Design review of the part built by this model. Coordinates are the model's own, in mm. A direction names the side the tool comes from. Round coordinates to 2 decimals unless told otherwise and drop trailing zeros. Order: outer loops, then holes, each group sorted by start corner. A loop starts at its lowest first (then second) coordinate and runs counter-clockwise, first axis right, second up.
from build123d import *

# Parameters (mm, degrees)
BOSS_EXTRUDE1_DEPTH       = 15.875
BOSS_EXTRUDE1_START       = -16.6878
BOSS_EXTRUDE1_2_OUTLINE_W = 13.242442679
BOSS_EXTRUDE1_2_OUTLINE_H = 1.4224
BOSS_EXTRUDE1_2_DEPTH     = 16.6878
BOSS_EXTRUDE2_START       = 15.875
BOSS_EXTRUDE2_DEPTH       = 15.875
SKETCH3_W                 = 13.242442679
SKETCH3_H                 = 1.4224
BOSS_EXTRUDE3_DEPTH       = 7.5311
SKETCH4_W                 = 13.242442679
SKETCH4_H                 = 1.4224
BOSS_EXTRUDE4_DEPTH       = 7.5311
CUT_EXTRUDE1_DEPTH        = 38.226845626
CUT_EXTRUDE2_DEPTH        = 38.226845626
CUT_EXTRUDE3_DEPTH        = 38.226845626
CUT_EXTRUDE4_DEPTH        = 38.226845626
SKETCH9_W                 = 4.6228
SKETCH9_H                 = 4.6228
CUT_EXTRUDE5_DEPTH        = 38.429132244
SKETCH10_W                = 4.6228
SKETCH10_H                = 4.6228
CUT_EXTRUDE6_DEPTH        = 38.429132244
SKETCH11_W                = 4.6228
SKETCH11_H                = 4.6228
CUT_EXTRUDE7_DEPTH        = 38.429132244
SKETCH12_W                = 4.6228
SKETCH12_H                = 4.6228
CUT_EXTRUDE8_DEPTH        = 38.429132244
SKETCH13_W                = 4.6228
SKETCH13_H                = 4.6228
CUT_EXTRUDE9_DEPTH        = 38.226845626
DRAFT1_ANGLE              = 45
DRAFT2_ANGLE              = 45
CHAMFER1_SIZE             = 2.24506403
SKETCH14_R                = 2.413
CUT_EXTRUDE10_DEPTH       = 2.54
LPATTERN1_COUNT           = 5
LPATTERN1_PITCH           = 12.7


with BuildPart() as part:
    # Boss-Extrude1: read off the stored shape, not the designer's step
    # Boss-Extrude1 outline → Boss-Extrude1 (new body)
    with BuildSketch(Plane(origin=(0, 0, -8.3439), x_dir=(-1, 0, 0), z_dir=(0, 0, -1))):
        with BuildLine():
            ThreePointArc((15.875, 0), (17.379950004, 5.616549878), (13.26835013, 1.504950004))
            Line((13.26835013, 1.504950004), (14.500184664, 2.216150004))
            ThreePointArc((14.500184664, 2.216150004), (16.668750004, 4.384715344), (15.875, 1.4224))
            Line((15.875, 1.4224), (-3.175, 1.4224))
            Line((-3.175, 1.4224), (-3.175, 0))
            Line((-3.175, 0), (15.875, 0))
        make_face()
    extrude(amount=BOSS_EXTRUDE1_DEPTH)

    # Boss-Extrude1 2 outline → Boss-Extrude1 2 (add)
    with BuildSketch(Plane(origin=(0, 0, -8.3439), x_dir=(-1, 0, 0), z_dir=(0, 0, -1)).offset(BOSS_EXTRUDE1_START)):
        with Locations((3.44622134, 0.7112)):
            Rectangle(BOSS_EXTRUDE1_2_OUTLINE_W, BOSS_EXTRUDE1_2_OUTLINE_H)
    extrude(amount=BOSS_EXTRUDE1_2_DEPTH)

    # Sketch2 → Boss-Extrude2 (add)
    with BuildSketch(Plane.XY.offset(8.3439).offset(BOSS_EXTRUDE2_START)):
        with BuildLine():
            Line((3.175, -6e-09), (-15.875, -6e-09))
            ThreePointArc((-15.875, -6e-09), (-17.379950004, 5.616549873), (-13.26835013, 1.504949999))
            Line((-13.26835013, 1.504949999), (-14.500184664, 2.216149999))
            ThreePointArc((-14.500184664, 2.216149999), (-16.668750004, 4.384715339), (-15.875, 1.422399994))
            Line((-15.875, 1.422399994), (3.175, 1.422399994))
            Line((3.175, 1.422399994), (3.175, -6e-09))
        make_face()
    extrude(amount=-BOSS_EXTRUDE2_DEPTH)

    # Sketch3 → Boss-Extrude3 (add)
    with BuildSketch(Plane(origin=(0, 0, -24.2189), x_dir=(-1, 0, 0), z_dir=(0, 0, -1))):
        with Locations((3.44622134, 0.7112)):
            Rectangle(SKETCH3_W, SKETCH3_H)
    extrude(amount=BOSS_EXTRUDE3_DEPTH)

    # Sketch4 → Boss-Extrude4 (add)
    with BuildSketch(Plane.XY.offset(24.2189)):
        with Locations((-3.44622134, 0.7112)):
            Rectangle(SKETCH4_W, SKETCH4_H)
    extrude(amount=BOSS_EXTRUDE4_DEPTH)

    # Sketch5 → Cut-Extrude1 (cut, through all)
    with BuildSketch(Plane(origin=(0, 1.4224, 0), x_dir=(-1, 0, 0), z_dir=(0, 1, 0))):
        Polygon((-3.175, -16.80493597), (-3.175, -21.29506403), (1.315128061, -16.80493597), align=None)
    extrude(amount=-CUT_EXTRUDE1_DEPTH, mode=Mode.SUBTRACT)

    # Sketch6 → Cut-Extrude2 (cut, through all)
    with BuildSketch(Plane(origin=(0, 1.4224, 0), x_dir=(-1, 0, 0), z_dir=(0, 1, 0))):
        Polygon((-3.175, -4.10493597), (-3.175, -8.59506403), (1.315128061, -8.59506403), align=None)
    extrude(amount=-CUT_EXTRUDE2_DEPTH, mode=Mode.SUBTRACT)

    # Sketch7 → Cut-Extrude3 (cut, through all)
    with BuildSketch(Plane(origin=(0, 1.4224, 0), x_dir=(-1, 0, 0), z_dir=(0, 1, 0))):
        Polygon((-3.175, 8.59506403), (-3.175, 4.10493597), (1.315128061, 8.59506403), align=None)
    extrude(amount=-CUT_EXTRUDE3_DEPTH, mode=Mode.SUBTRACT)

    # Sketch8 → Cut-Extrude4 (cut, through all)
    with BuildSketch(Plane(origin=(0, 1.4224, 0), x_dir=(-1, 0, 0), z_dir=(0, 1, 0))):
        Polygon((-3.175, 21.29506403), (-3.175, 16.80493597), (1.315128061, 16.80493597), align=None)
    extrude(amount=-CUT_EXTRUDE4_DEPTH, mode=Mode.SUBTRACT)

    # Sketch9 → Cut-Extrude5 (cut, through all)
    with BuildSketch(Plane.XZ):
        with Locations((-3.175, 25.4)):
            Rectangle(SKETCH9_W, SKETCH9_H)
    extrude(amount=-CUT_EXTRUDE5_DEPTH, mode=Mode.SUBTRACT)

    # Sketch10 → Cut-Extrude6 (cut, through all)
    with BuildSketch(Plane.XZ):
        with Locations((-3.175, 12.7)):
            Rectangle(SKETCH10_W, SKETCH10_H)
    extrude(amount=-CUT_EXTRUDE6_DEPTH, mode=Mode.SUBTRACT)

    # Sketch11 → Cut-Extrude7 (cut, through all)
    with BuildSketch(Plane.XZ):
        with Locations((-3.175, 0)):
            Rectangle(SKETCH11_W, SKETCH11_H)
    extrude(amount=-CUT_EXTRUDE7_DEPTH, mode=Mode.SUBTRACT)

    # Sketch12 → Cut-Extrude8 (cut, through all)
    with BuildSketch(Plane.XZ):
        with Locations((-3.175, -12.7)):
            Rectangle(SKETCH12_W, SKETCH12_H)
    extrude(amount=-CUT_EXTRUDE8_DEPTH, mode=Mode.SUBTRACT)

    # Sketch13 → Cut-Extrude9 (cut, through all)
    with BuildSketch(Plane(origin=(0, 1.4224, 0), x_dir=(-1, 0, 0), z_dir=(0, 1, 0))):
        with Locations((3.175, -25.4)):
            Rectangle(SKETCH13_W, SKETCH13_H)
    extrude(amount=-CUT_EXTRUDE9_DEPTH, mode=Mode.SUBTRACT)

    # Draft1
    draft1_faces = [part.faces().sort_by_distance(p)[0] for p in [
        (0.92993597, 0.7112, -8.59506403),
        (0.92993597, 0.711199999, -16.80493597),
    ]]
    draft(draft1_faces, Plane(origin=(3.175, 0, 31.75), x_dir=(0, 0, 1), z_dir=(1, 0, 0)), DRAFT1_ANGLE)

    # Draft2
    draft2_faces = [part.faces().sort_by_distance(p)[0] for p in [
        (0.92993597, 0.7112, 16.80493597),
        (0.92993597, 0.711199997, 8.59506403),
    ]]
    draft(draft2_faces, Plane(origin=(3.175, 0, 31.75), x_dir=(0, 0, 1), z_dir=(1, 0, 0)), DRAFT2_ANGLE)

    # Chamfer1
    chamfer1_edges = [part.edges().sort_by_distance(p)[0] for p in [
        (3.175, 0.7112, 31.75),
        (-10.067442679, 0.7112, 31.75),
        (3.175, 0.7112, -31.75),
        (-10.067442679, 0.7112, -31.75),
    ]]
    chamfer(chamfer1_edges, length=CHAMFER1_SIZE)

    # Sketch14 → Cut-Extrude10 (cut)
    with BuildSketch(Plane(origin=(0, 1.4224, 0), x_dir=(1, 0, 0), z_dir=(0, 1, 0))):
        with Locations((-3.175, -25.4)):
            Circle(SKETCH14_R)
    cut_extrude10 = extrude(amount=-CUT_EXTRUDE10_DEPTH, mode=Mode.SUBTRACT)

    # LPattern1: Cut-Extrude10 ×5
    with Locations(*[(0, 0, -i * LPATTERN1_PITCH) for i in range(1, LPATTERN1_COUNT)]):
        add(cut_extrude10, mode=Mode.SUBTRACT)


solid = part.part
1) To check wall thickness, follow line 1 along Z through (x, y) = (-2, 0.5); line 2 along Z through (x, y) = (-17.75, 2.5); line 3 along Y through (x, z) = (-1.5, 18.5). State the ranges of each line that lie inside material, in increasing order.
Results:
line 1: z = -31.75 to -27.71, -23.09 to -15.01, -10.39 to -2.31, 2.31 to 10.39, 15.01 to 23.09, 27.71 to 31.75
line 2: z = -24.22 to -8.34, 8.34 to 24.22
line 3: y = 0 to 1.42
2) Clearance check with flat-ended pins moving along their axes: P1, Ø3, axis at y = 1, z = -2, coming from the -X side; P2, Ø1.1, axis at y = 0.5, z = 14, coming from the -X side; P3, Ø3, axis at x = -12, z = 2, coming from the +Y side; P4, Ø1.6, axis at y = 0.5, z = 11.5, coming from the -X side. State where each tip first meets the part, or that it passes through.
Results:
P1: stops at x = -10.07
P2: stops at x = -18.16
P3: passes through
P4: stops at x = -18.35
3) For faces 1 (the face through (3.175, 1, -25)), 2 (the face through (2.04, 0.72, 7.46)), 3 (the face through (-13.88, 1.86, -16.17)), 4 (the face through (-0.864, 1, 1)), list the 3-axis set-ups (+Z, -Z, +X, -X, +Y, -Y) from which the entire face can be reached by the end or side of a thin tool; tool diameter is ignored.
Results:
face 1: +Z, -Z, +X, +Y, -Y
face 2: +X, +Y, -Y
face 3: +Z, -Z
face 4: +Y, -Y
4) Take a section at C-C on y = 4. Give the boundary of the cut face in (x, z), plus the area to 3 significant figures.
Results:
outline: (-18.72, -24.22) - (-17.12, -24.22) - (-17.12, -8.34) - (-18.72, -8.34) - close; (-18.72, 8.34) - (-17.12, 8.34) - (-17.12, 24.22) - (-18.72, 24.22) - close; (-14.63, -24.22) - (-13.03, -24.22) - (-13.03, -8.34) - (-14.63, -8.34) - close; (-14.63, 8.34) - (-13.03, 8.34) - (-13.03, 24.22) - (-14.63, 24.22) - close
area: 102 mm2
5) Take a section at D-D on z = -17.5. Give the boundary of the cut face in (x, y) (1 decimal), plus the area to 3 significant figures.
Results:
outline: (-15.9, 0) - (2.5, 0) - (2.5, 1.4) - (-15.9, 1.4) arc R1.6 cw (long way) to (-14.5, 2.2) - (-13.3, 1.5) arc R3 ccw (long way) to start
area: 43.2 mm2
6) The part is to be moulded in two halves that separate along Y. For faces 5 (the face through (-3.185, 0.721, -22.987)), 6 (the face through (-13.88, 1.86, 16.39)), say which applies: released by +Y, released by -Y, zero draft, split by the parting line, or undercut.
Results:
face 5: zero draft
face 6: undercut
7) Take a section at B-B on x = -16.75. Give the boundary of the cut face in (y, z), plus the area to 3 significant figures.
Results:
outline: (0.13, -24.22) - (1.69, -24.22) - (1.69, -8.34) - (0.13, -8.34) - close; (0.13, 8.34) - (1.69, 8.34) - (1.69, 24.22) - (0.13, 24.22) - close; (4.33, -24.22) - (5.89, -24.22) - (5.89, -8.34) - (4.33, -8.34) - close; (4.33, 8.34) - (5.89, 8.34) - (5.89, 24.22) - (4.33, 24.22) - close
area: 98.8 mm2
8) Take a section at A-A on x = -4.75. Give the boundary of the cut face in (y, z), plus the area to 3 significant figures.
Results:
outline: (0, -31.75) - (1.42, -31.75) - (1.42, -27.71) - (0, -27.71) - close; (0, -23.09) - (1.42, -23.09) - (1.42, -15.01) - (0, -15.01) - close; (0, -10.39) - (1.42, -10.39) - (1.42, -2.31) - (0, -2.31) - close; (0, 2.31) - (1.42, 2.31) - (1.42, 10.39) - (0, 10.39) - close; (0, 15.01) - (1.42, 15.01) - (1.42, 23.09) - (0, 23.09) - close; (0, 27.71) - (1.42, 27.71) - (1.42, 31.75) - (0, 31.75) - close
area: 57.4 mm2
